from build123d import *

# Parameters (mm, degrees)
SKETCH_W        = 30
SKETCH_H        = 20
PAD_DEPTH       = 13
SKETCH001_R     = 1
POCKET_DEPTH    = 13.001
SKETCH002_R     = 4
POCKET001_DEPTH = 8
SKETCH003_R     = 2.1
POCKET002_DEPTH = 20.001


with BuildPart() as part:
    # Sketch → Pad (new body)
    with BuildSketch(Plane.XY):
        Rectangle(SKETCH_W, SKETCH_H)
    extrude(amount=PAD_DEPTH)

    # Sketch001 (on Face6 of Pad) → Pocket (cut, through all)
    with BuildSketch(Plane.XY.offset(13)):
        with Locations((-11.25, 7.25)):
            Circle(SKETCH001_R)
        with Locations((0.25, 7.25)):
            Circle(SKETCH001_R)
        with Locations((-11.25, -4.25)):
            Circle(SKETCH001_R)
        with Locations((0.25, -4.25)):
            Circle(SKETCH001_R)
        with Locations((11.75, 7.25)):
            Circle(SKETCH001_R)
        with Locations((11.75, -4.25)):
            Circle(SKETCH001_R)
    extrude(amount=-POCKET_DEPTH, mode=Mode.SUBTRACT)

    # Sketch002 (on Face4 of Pocket) → Pocket001 (cut)
    with BuildSketch(Plane(origin=(0, 0, 0), x_dir=(1, 0, 0), z_dir=(0, 0, -1))):
        with Locations((-5.5, -1.5)):
            Circle(SKETCH002_R)
    extrude(amount=-POCKET001_DEPTH, mode=Mode.SUBTRACT)

    # Sketch003 (on Face1 of Pocket001) → Pocket002 (cut, through all)
    with BuildSketch(Plane(origin=(0, 10, 0), x_dir=(-1, 0, 0), z_dir=(0, 1, 0))):
        with Locations((5.5, 6.5)):
            Circle(SKETCH003_R)
        with Locations((-6, 6.5)):
            Circle(SKETCH003_R)
    extrude(amount=-POCKET002_DEPTH, mode=Mode.SUBTRACT)


solid = part.part
The listing builds one solid part. Answer for the finished solid, in the listing's coordinates (mm). A direction names the side the tool comes from. Coordinates: 2 decimals unless noted, no trailing zeros. Write each loop counter-clockwise with the first axis right and the second up, starting at its lowest first coordinate (ties: lowest second). Pieces come first, ordered by that corner, then holes. Notation, with made-up numbers: M 13,1 L 56,1 A21 ccw 56,28 Z; hole C 34,54 d11. An arc over 180 degrees is marked long. Put each result on its own line as item: value. Start each with the question number.
1. For a pull along Z with two mould halves and no side action, classify faces 3 (the flat face through (-3, 1, 8)), 4 (the cylindrical face through (6.273, 0.14, 8.582)), 5 (the flat face through (0, 10, 6)) as pulls with the +Z half, pulls with the -Z half, needs draft (parallel to the pull), parting line crosses it, or undercut.
2. A cutting plane is placed at B-B on z = 6.5. Count the separate pieces of the cut face and the enclosed holes in it, then the cut area to 3 significant figures.
3. A cutting plane is placed at C-C on y = 1.5. Write down the section's boundary in (x, z), then the cut area to 3 significant figures.
4. Which of the six approach directions +Z, -Z, +X, -X, +Y, -Y give full straight-line access (tool end or side, diameter ignored) to faces 1 (the cylindrical face through (-11.987, -3.574, 6.591)), 2 (the flat face through (-8, 1, 8))?
5. Consider line 1 (Y direction, x = 0.25, z = 3.75); line 2 (Z direction, x = 6, y = 1); line 3 (X direction, y = 1.5, z = 2.25). Determine where each line is inside the solid, lowest interval first. Write a range as from..to.
6. A cutting plane is placed at A-A on y = 7.25. Write down the section's boundary in (x, z), then the cut area to 3 significant figures.
7. A cutting plane is placed at D-D on z = 2.75. Write down the section's boundary in (x, y), then the cut area to 3 significant figures.
Resolved:
1. face 3: pulls with the -Z half
1. face 4: undercut
1. face 5: needs draft
2. separate pieces: 3
2. enclosed holes: 6
2. area: 395 mm2
3. outline: M -15,0 L -9.5,0 L -9.5,8 L -6.97,8 A2.1 cw -4.03,8 L -1.5,8 L -1.5,0 L 15,0 L 15,13 L -15,13 Z; hole C 6,6.5 d4.2
3. area: 311 mm2
4. face 1: +Z, -Z
4. face 2: -Z
5. line 1: y = -10..-5.25, -3.25..6.25, 8.25..10
5. line 2: z = 0..4.4, 8.6..13
5. line 3: x = -15..-9.5, -1.5..15
6. outline: M -15,0 L -12.25,0 L -12.25,13 L -15,13 Z; M -10.25,0 L -0.75,0 L -0.75,13 L -10.25,13 Z; M 1.25,0 L 10.75,0 L 10.75,13 L 1.25,13 Z; M 12.75,0 L 15,0 L 15,13 L 12.75,13 Z; hole C -5.5,6.5 d4.2; hole C 6,6.5 d4.2
6. area: 284 mm2
7. outline: M -15,-10 L 15,-10 L 15,10 L -15,10 Z; hole C -11.25,-4.25 d2; hole C -11.25,7.25 d2; hole C -5.5,1.5 d8; hole C 0.25,-4.25 d2; hole C 0.25,7.25 d2; hole C 11.75,-4.25 d2; hole C 11.75,7.25 d2
7. area: 531 mm2
